Can you work these out from the model? Positions are in its coordinate system, mm. A direction names the side the tool comes from. Give positions to 0.01 mm unless a question says otherwise; leave off trailing zeros. Write each loop counter-clockwise with the first axis right and the second up, starting at its lowest first coordinate (ties: lowest second). Pieces come first, ordered by that corner, then holes. Notation, with made-up numbers: (89, -5.75) -> (106, -5.75) arc R24 ccw to (106, 27.25) -> close; hole circle Ø11 at (69, 46.5). An arc over 180 degrees is marked (long way). One line per item, written item: value.
from build123d import *

# Parameters (mm, degrees)
SKETCH2_W           = 125.512132551
SKETCH2_H           = 55
SKETCH2_R           = 7
BOSS_EXTRUDE1_DEPTH = 7
FILLET4_R           = 20
SKETCH5_R           = 2.025
CUT_EXTRUDE1_DEPTH  = 10
SKETCH6_R           = 2.025
CUT_EXTRUDE2_DEPTH  = 33
SKETCH7_R           = 3.125
CUT_EXTRUDE3_DEPTH  = 4.7
SKETCH8_R           = 2.025
CUT_EXTRUDE4_DEPTH  = 7


with BuildPart() as part:
    # Sketch2 → Boss-Extrude1 (new body)
    with BuildSketch(Plane(origin=(0, 0, 0), x_dir=(1, 0, 0), z_dir=(0, 1, 0))):
        with Locations((82.945127875, 24.3964427)):
            Rectangle(SKETCH2_W, SKETCH2_H)
        with Locations(Location((36.189061599, 31.8964427, 0), (0, 0, 270))):
            Circle(SKETCH2_R, mode=Mode.SUBTRACT)
        with Locations(Location((129.70119415, 31.8964427, 0), (0, 0, 270))):
            Circle(SKETCH2_R, mode=Mode.SUBTRACT)
    extrude(amount=BOSS_EXTRUDE1_DEPTH)

    # Fillet4
    fillet4_edges = [part.edges().sort_by_distance(p)[0] for p in [
        (145.70119415, 3.5, -51.8964427),
        (20.189061599, 3.5, -51.8964427),
    ]]
    fillet(fillet4_edges, radius=FILLET4_R)

    # Sketch5 → Cut-Extrude1 (cut)
    with BuildSketch(Plane(origin=(0, 7, 0), x_dir=(1, 0, 0), z_dir=(0, 1, 0))):
        with Locations(Location((109.81119415, 32.1464427, 0), (0, 0, 270))):
            Circle(SKETCH5_R)
    extrude(amount=-CUT_EXTRUDE1_DEPTH, mode=Mode.SUBTRACT)

    # Sketch6 → Cut-Extrude2 (cut)
    with BuildSketch(Plane(origin=(0, 7, 0), x_dir=(1, 0, 0), z_dir=(0, 1, 0))):
        with Locations(Location((28.189061599, 39.8964427, 0), (0, 0, 270))):
            Circle(SKETCH6_R)
        with Locations(Location((44.189061599, 39.8964427, 0), (0, 0, 270))):
            Circle(SKETCH6_R)
        with Locations(Location((44.189061599, 23.8964427, 0), (0, 0, 270))):
            Circle(SKETCH6_R)
        with Locations(Location((28.189061599, 23.8964427, 0), (0, 0, 270))):
            Circle(SKETCH6_R)
    extrude(amount=-CUT_EXTRUDE2_DEPTH, mode=Mode.SUBTRACT)

    # Sketch7 → Cut-Extrude3 (cut)
    with BuildSketch(Plane.XY.offset(3.1035573)):
        with Locations((25.189061599, 3.5)):
            Circle(SKETCH7_R)
        with Locations((130.70119415, 3.5)):
            Circle(SKETCH7_R)
        with Locations((82.945127875, 3.5)):
            Circle(SKETCH7_R)
    extrude(amount=-CUT_EXTRUDE3_DEPTH, mode=Mode.SUBTRACT)

    # Sketch8 → Cut-Extrude4 (cut)
    with BuildSketch(Plane(origin=(0, 7, 0), x_dir=(1, 0, 0), z_dir=(0, 1, 0))):
        with Locations(Location((56.514656449, 46.8964427, 0), (0, 0, 270))):
            Circle(SKETCH8_R)
    extrude(amount=-CUT_EXTRUDE4_DEPTH, mode=Mode.SUBTRACT)


solid = part.part
1) I need wall thicknesses on L1, parallel to X at y = 4.5, z = -31; L2, parallel to X at y = 6.25, z = -36.5; L3, parallel to X at y = 5.5, z = -0.5. Which ranges of each line are inside material? Lowest first, please.
Answer list:
L1: x = 20.19 to 29.25, 43.13 to 108.14, 111.48 to 122.76, 136.64 to 145.7
L2: x = 20.73 to 30.92, 41.46 to 124.43, 134.97 to 145.16
L3: x = 20.19 to 22.79, 27.59 to 80.54, 85.35 to 128.3, 133.1 to 145.7
2) We'd pull the mould along Y, two halves only. Please class faces 3 (the face through (82, 0, -25)), 4 (the face through (139.69, 3.55, -46.19)), 5 (the face through (82, 7, -25)), 6 (the face through (25, 4, -1.596)): released by +Y, released by -Y, zero draft, split by the parting line, or undercut.
Answer list:
face 3: released by -Y
face 4: zero draft
face 5: released by +Y
face 6: undercut
3) If we section it at C-C (y = 3.5): State how many separate pieces and enclosed holes the cut face has, and give its area (3 significant figures).
Answer list:
separate pieces: 1
enclosed holes: 8
area: 6,260 mm^2
4) For faces 1 (the face through (83, 4, -1.596)), 2 (the face through (145.701, 3, -14)), which set-ups out of +Z, -Z, +X, -X, +Y, -Y let a thin tool reach every point of the face, with its end or its side?
Answer list:
face 1: +Z
face 2: +Z, -Z, +X, +Y, -Y
5) If we section it at A-A (x = 124): Write out the boundary of the cut face in (y, z), and give its area (3 significant figures).
Answer list:
outline: (0, -51.9) -> (7, -51.9) -> (7, -35.96) -> (0, -35.96) -> close; (0, -27.83) -> (7, -27.83) -> (7, 3.1) -> (0, 3.1) -> close
area: 328 mm^2
6) If we section it at D-D (z = -28.5): Write out the boundary of the cut face in (x, y).
Answer list:
outline: (20.19, 0) -> (30.07, 0) -> (30.07, 7) -> (20.19, 7) -> close; (42.31, 0) -> (123.58, 0) -> (123.58, 7) -> (42.31, 7) -> close; (135.82, 0) -> (145.7, 0) -> (145.7, 7) -> (135.82, 7) -> close
7) If we section it at B-B (z = -40): Write out the boundary of the cut face in (x, y).
Answer list:
outline: (21.9, 0) -> (26.17, 0) -> (26.17, 7) -> (21.9, 7) -> close; (30.21, 0) -> (42.17, 0) -> (42.17, 7) -> (30.21, 7) -> close; (46.21, 0) -> (143.99, 0) -> (143.99, 7) -> (46.21, 7) -> close
8) Will this pin go through, and if not, where does the flat tip stop? pin 1 (4 mm diameter, centred on x = 82.95, y = 3.5, fed in from +Z).
Answer list:
pin 1: stops at z = -1.6
